```python
from build123d import *

# Parameters (mm, degrees)
SKETCH1_W                 = 42
SKETCH1_H                 = 42
BOSS_EXTRUDE2_DEPTH       = 30
SHELL1_T                  = 4
SKETCH3_R                 = 3.5
CUT_EXTRUDE1_DEPTH        = 30
SKETCH2_R                 = 6.75
CUT_EXTRUDE2_DEPTH        = 30
SKETCH5_R                 = 4
BOSS_EXTRUDE3_DEPTH       = 34
F_6_32_TAPPED_HOLE6_D     = 2.7051
F_6_32_TAPPED_HOLE6_DEPTH = 10.97
F_6_32_TAPPED_HOLE6_TIP   = 0.81269403
FILLET3_R                 = 10


with BuildPart() as part:
    # Sketch1 → Boss-Extrude2 (new body)
    with BuildSketch(Plane(origin=(0, 0, 0), x_dir=(1, 0, 0), z_dir=(0, 1, 0))):
        Rectangle(SKETCH1_W, SKETCH1_H)
    extrude(amount=BOSS_EXTRUDE2_DEPTH)

    # Shell1
    shell1_openings = [part.faces().sort_by_distance(p)[0] for p in [
        (0, 30, 0),
    ]]
    offset(amount=SHELL1_T, openings=shell1_openings, kind=Kind.INTERSECTION)

    # Sketch3 → Cut-Extrude1 (cut)
    with BuildSketch(Plane(origin=(0, 0, 0), x_dir=(0, 0, -1), z_dir=(1, 0, 0))):
        with Locations((0, 17)):
            Circle(SKETCH3_R)
    extrude(amount=-CUT_EXTRUDE1_DEPTH, mode=Mode.SUBTRACT)

    # Sketch2 → Cut-Extrude2 (cut)
    with BuildSketch(Plane(origin=(0, -4, 0), x_dir=(-1, 0, 0), z_dir=(0, -1, 0))):
        with Locations(Location((0, 0, 0), (0, 0, 90))):
            Circle(SKETCH2_R)
    extrude(amount=-CUT_EXTRUDE2_DEPTH, mode=Mode.SUBTRACT)

    # Sketch5 → Boss-Extrude3 (add)
    with BuildSketch(Plane(origin=(0, -4, 0), x_dir=(-1, 0, 0), z_dir=(0, -1, 0))):
        with Locations((20, -20)):
            Circle(SKETCH5_R)
        with Locations((-20, -20)):
            Circle(SKETCH5_R)
        with Locations((-20, 20)):
            Circle(SKETCH5_R)
        with Locations((20, 20)):
            Circle(SKETCH5_R)
    extrude(amount=-BOSS_EXTRUDE3_DEPTH)

    # #6-32 Tapped Hole6
    with Locations(Plane(origin=(-20, 30, -20), x_dir=(0, 0, 1), z_dir=(0, 1, 0))):
        with Locations((0, 0), (0, 40), (40, 40), (40, 0)):
            Hole(F_6_32_TAPPED_HOLE6_D / 2, depth=F_6_32_TAPPED_HOLE6_DEPTH)
            with Locations((0, 0, -(F_6_32_TAPPED_HOLE6_DEPTH + F_6_32_TAPPED_HOLE6_TIP / 2))):  # 118° drill point
                Cone(0, F_6_32_TAPPED_HOLE6_D / 2, F_6_32_TAPPED_HOLE6_TIP, mode=Mode.SUBTRACT)

    # Fillet3
    fillet3_edges = [part.edges().sort_by_distance(p)[0] for p in [
        (25, 13, 25),
        (-25, 13, 25),
        (-25, 13, -25),
        (25, 13, -25),
    ]]
    fillet(fillet3_edges, radius=FILLET3_R)


solid = part.part
```
Could you check a few things on this model? Use its own coordinates, in mm. A direction names the side the tool comes from. Coordinates: 2 decimals unless noted, no trailing zeros. Order: outer loops, then holes, each group sorted by start corner. A loop starts at its lowest first (then second) coordinate and runs counter-clockwise, first axis right, second up. Notation, with made-up numbers: M 58,70.5 L 65,70.5 A23 cw 65,91.5 Z; hole C -32.75,2.25 d3. An arc over 180 degrees is marked long. Use a Markdown table: item, result. Add a question column.
Q1. We'd pull the mould along X, two halves only. Please class faces 3 (the flat face through (0, 13, -25)), 4 (the cylindrical face through (-22.15, 12.76, 21.99)), 5 (the cylindrical face through (21.99, 13.24, 22.15)), 6 (the cylindrical face through (-18.86, 24.44, -20.73)): pulls with the +X half, pulls with the -X half, needs draft (parallel to the pull), parting line crosses it, or undercut.
Q2. I want a section at A-A on z = 0. List the corners of the cut face in (x, y) for me, then the cut area to 3 significant figures.
Q3. I'm going to push flat-ended pins straight in: pin 1 (2 mm diameter, centred on x = -1, z = -13.5, fed in from +Y); pin 2 (2.5 mm diameter, centred on x = 20, z = -20, fed in from +Y); pin 3 (6.5 mm diameter, centred on y = 17, z = 0, fed in from -X). Where does each tip first touch, or does it pass through?
Q4. Which directions (+Z, -Z, +X, -X, +Y, -Y) give clear straight access to the entire face, cutting with the end or side of a thin tool? Please do faces 1 (the cylindrical face through (21.14, 24.44, 19.27)), 2 (the flat face through (25, 13, 0)).
Q5. I want a section at B-B on x = -1.5. List the corners of the cut face in (y, z) for me, then the cut area to 3 significant figures.
Q6. If I drill on L1, parallel to Z at x = 4, y = 5; L2, parallel to X at y = -1, z = 0; L3, parallel to X at y = 28.5, z = -19.5, over which ranges is the centre line in solid material (lowest first)?
Q7. I want a section at C-C on y = 5.5. List the corners of the cut face in (x, z) for me, then the cut area to 3 significant figures.
Q8. I want a section at D-D on y = 24.5. List the corners of the cut face in (x, z) for me, then the cut area to 3 significant figures.
Checked values:
| question | item | result |
|---|---|---|
| 1 | face 3 | needs draft |
| 1 | face 4 | pulls with the -X half |
| 1 | face 5 | pulls with the +X half |
| 1 | face 6 | undercut |
| 2 | outline | M -25,-4 L -6.75,-4 L -6.75,0 L -21,0 L -21,13.5 L -25,13.5 Z; M -25,20.5 L -21,20.5 L -21,30 L -25,30 Z; M 6.75,-4 L 25,-4 L 25,30 L 21,30 L 21,0 L 6.75,0 Z |
| 2 | area | 358 mm² |
| 3 | pin 1 | y = 0 |
| 3 | pin 2 | y = 18.97 |
| 3 | pin 3 | x = 21 |
| 4 | face 1 | +Y |
| 4 | face 2 | +Z, -Z, +X, +Y, -Y |
| 5 | outline | M -4,-25 L 30,-25 L 30,-21 L 0,-21 L 0,-6.58 L -4,-6.58 Z; M -4,6.58 L 0,6.58 L 0,21 L 30,21 L 30,25 L -4,25 Z |
| 5 | area | 387 mm² |
| 6 | L1 | -25 to -21, 21 to 25 |
| 6 | L2 | -25 to -6.75, 6.75 to 25 |
| 6 | L3 | -23.93 to -21.26, -18.74 to -16.03, 16.03 to 18.74, 21.26 to 23.93 |
| 7 | outline | M -25,-15 A10 ccw -15,-25 L 15,-25 A10 ccw 25,-15 L 25,15 A10 ccw 15,25 L -15,25 A10 ccw -25,15 Z; hole M -21,-16.13 A4 cw -16.13,-21 L 16.13,-21 A4 cw 21,-16.13 L 21,16.13 A4 cw 16.13,21 L -16.13,21 A4 cw -21,16.13 Z |
| 7 | area | 736 mm² |
| 8 | outline | M -25,-15 A10 ccw -15,-25 L 15,-25 A10 ccw 25,-15 L 25,15 A10 ccw 15,25 L -15,25 A10 ccw -25,15 Z; hole C -20,-20 d2.71; hole C -20,20 d2.71; hole M -21,-16.13 A4 cw -16.13,-21 L 16.13,-21 A4 cw 21,-16.13 L 21,16.13 A4 cw 16.13,21 L -16.13,21 A4 cw -21,16.13 Z; hole C 20,-20 d2.71; hole C 20,20 d2.71 |
| 8 | area | 713 mm² |
